Design review of the part built by this model. Coordinates are the model's own, in mm. Face numbers are marked on the shaded views. A direction names the side the tool comes from. Round coordinates to 2 decimals unless told otherwise and drop trailing zeros. Order: outer loops, then holes, each group sorted by start corner. A loop starts at its lowest first (then second) coordinate and runs counter-clockwise, first axis right, second up. Notation, with made-up numbers: M 44,-11 L 99,-11 A20 ccw 99,23 Z; hole C 46,6.25 d4. An arc over 180 degrees is marked long. Write each question's results on one line, items separated by ' | '. Start each with the question number.
Item 1: Clearance check with flat-ended pins moving along their axes: pin 1 (3 mm diameter, centred on y = 21.5, z = 10.5, fed in from -X); pin 2 (1 mm diameter, centred on y = 11.5, z = 11.5, fed in from +X); pin 3 (2 mm diameter, centred on x = -33, z = 19.5, fed in from -Y); pin 4 (8.5 mm diameter, centred on x = -35.5, z = 16.5, fed in from +Y). State where each tip first meets the part, or that it passes through.
Item 2: Wall thickness on line 1 (Y direction, x = 0, z = 11.25); line 2 (X direction, y = -4.5, z = 20.25); line 3 (Y direction, x = -28.5, z = 4.25): over which ranges is each line inside the solid? List them lowest first. Write a range as [from, to].
Item 3: Take a section at A-A, the plane x = 0. Write out the cut boundary in (y, z), plus the area to 3 significant figures.
Item 4: Take a section at B-B, the plane z = 23.5. Write out the cut boundary in (x, y) (1 decimal), plus the area to 3 significant figures.
Item 5: Take a section at C-C, the plane y = -16.5. Write out the cut boundary in (x, z).
Item 6: Machinability: for the marked faces 1 and 2, which of the approach directions +Z, -Z, +X, -X, +Y, -Y give a long, thin tool a straight path to every point of the face, cutting with its end or side? Answer none if there is none.
Item 7: The part is to be moulded in two halves that separate along X. For the marked faces 3, 4, 5 and 6, say which applies: +X half, -X half, draft (parallel to the pull), parting line (faces both ways), or undercut.
Item 8: Take a section at D-D, the plane y = 0. Write out the cut boundary in (x, z), plus the area to 3 significant figures.
```python
from build123d import *

# Parameters (mm, degrees)
F1_DEPTH       = 25.4
F3_D           = 3.3
F3_CBORE_D     = 6.5
F3_CBORE_DEPTH = 3
F5_DEPTH       = 5


with BuildPart() as f1:
    # F0 (on Top) → F1 (new body)
    with BuildSketch(Plane.XY):
        with BuildLine():
            ThreePointArc((-27.8767053979, 1.8796), (27.94, 0), (-27.8767053979, -1.8796))
            Line((-27.8767053979, -1.8796), (-29.4676154463, -1.8796))
            Line((-29.4676154463, -1.8796), (-38.3576154463, -1.8796))
            Line((-38.3576154463, -1.8796), (-38.3576154463, -10.7696))
            Line((-38.3576154463, -10.7696), (-29.4676154463, -10.7696))
            Line((-29.4676154463, -10.7696), (-27.4934350726, -10.7696))
            ThreePointArc((-27.4934350726, -10.7696), (29.5275, 0), (-27.4934350726, 10.7696))
            Line((-27.4934350726, 10.7696), (-29.4676154463, 10.7696))
            Line((-29.4676154463, 10.7696), (-38.3576154463, 10.7696))
            Line((-38.3576154463, 10.7696), (-38.3576154463, 1.8796))
            Line((-38.3576154463, 1.8796), (-29.4676154463, 1.8796))
            Line((-29.4676154463, 1.8796), (-27.8767053979, 1.8796))
        make_face()
    extrude(amount=F1_DEPTH)

    # F3 (through all)
    with Locations(Plane.XZ.offset(10.7696)):
        with Locations((-32.8522585332, 18.9988464117)):
            CounterBoreHole(F3_D / 2, F3_CBORE_D / 2, F3_CBORE_DEPTH)

    # F4 (on face) → F5 (cut)
    with BuildSketch(Plane(origin=(0, 10.7696, 0), x_dir=(-1, 0, 0), z_dir=(0, 1, 0))):
        Polygon((34.6081861546, 15.6860156038), (36.599217982, 18.8631089351), (34.8432903606, 22.175939743), (31.0963309118, 22.3116772196), (29.1052990845, 19.1345838883), (30.8612267059, 15.8217530804), align=None)
    extrude(amount=-F5_DEPTH, mode=Mode.SUBTRACT)


solid = f1.part
```
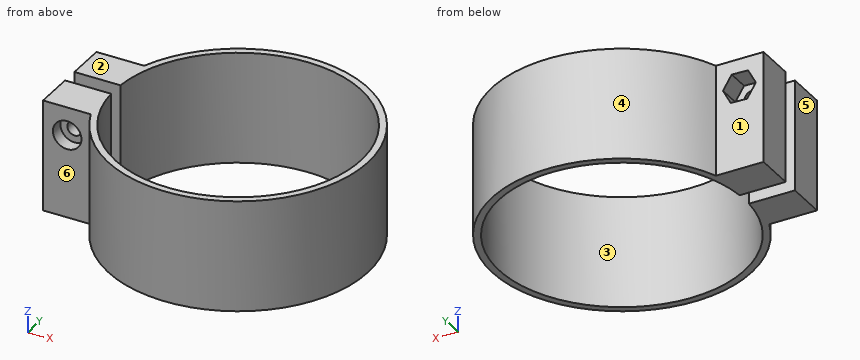
Results list:
1) pin 1: x = -21.72 | pin 2: x = 27.4 | pin 3: through | pin 4: y = 10.77
2) line 1: [-29.53, -27.94], [27.94, 29.53] | line 2: [-38.36, -33.93], [-31.78, -27.58], [27.58, 29.18] | line 3: [-10.77, -1.88], [1.88, 10.77]
3) outline: M -29.53,0 L -27.94,0 L -27.94,25.4 L -29.53,25.4 Z; M 27.94,0 L 29.53,0 L 29.53,25.4 L 27.94,25.4 Z | area: 80.6 mm²
4) outline: M -38.4,-10.8 L -27.5,-10.8 A29.5 ccw long -27.5,10.8 L -38.4,10.8 L -38.4,1.9 L -27.9,1.9 A27.9 cw long -27.9,-1.9 L -38.4,-1.9 Z | area: 452 mm²
5) outline: M -24.49,0 L -22.55,0 L -22.55,25.4 L -24.49,25.4 Z; M 22.55,0 L 24.49,0 L 24.49,25.4 L 22.55,25.4 Z
6) face 1: +Z, -Z, -X, +Y | face 2: +Z, +X, -X, +Y, -Y
7) face 3: undercut | face 4: parting line | face 5: -X half | face 6: draft
8) outline: M 27.94,0 L 29.53,0 L 29.53,25.4 L 27.94,25.4 Z | area: 40.3 mm²
